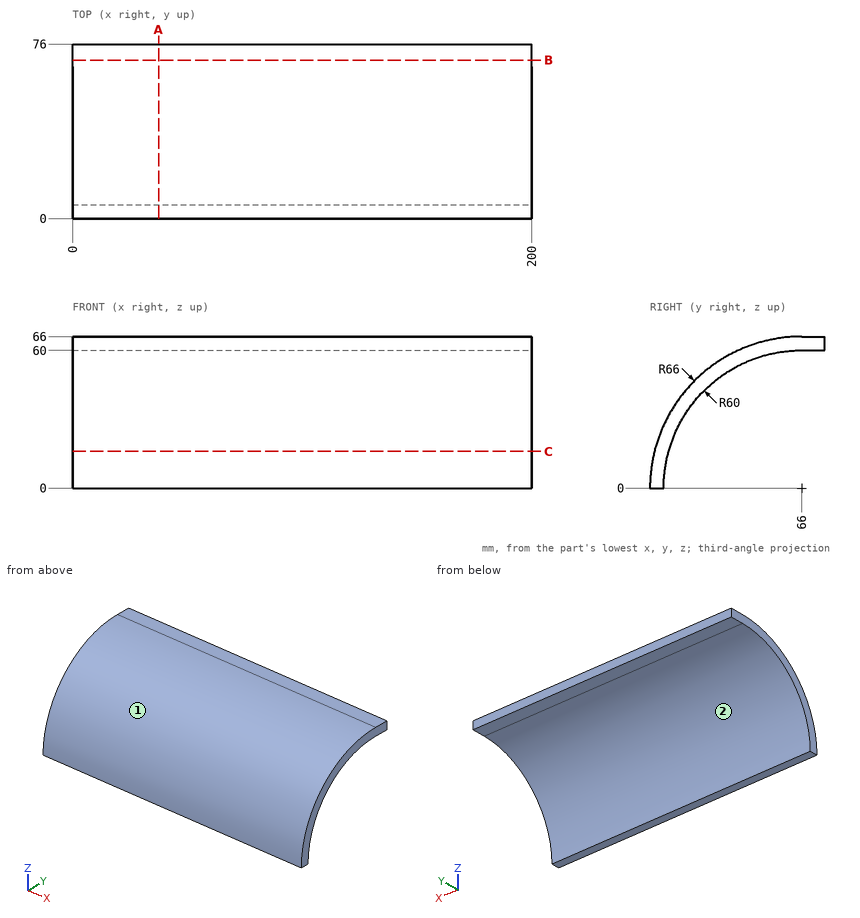
Verification items for this drawing (mm, ordinates from the low corner). Coordinates: 2 decimals unless noted, no trailing zeros. Loops run counter-clockwise (first coordinate to the right, second up) from the corner with the lowest first, then second, coordinate; pieces in that order, holes last. Notation, with made-up numbers: (83, 73) - (129, 73) arc R37 ccw to (129, 111) - close; hole circle Ø2 at (3.5, 13.5). An arc over 180 degrees is marked (long way). Use one line per item in the form item = value. Start each with the question number.
Item 1: Mould release check, pull along Z, two halves, no side actions. Record for the marked faces 1 and 2: +Z half, -Z half, draft (parallel to the pull), parting line (faces both ways), or undercut.
Item 2: Section check A-A, the plane x = 37.5. Enter the section's corners in (y, z).
Item 3: Thickness scan on probe 1 along Z at (x, y) = (176, 64); probe 2 along Z at (x, y) = (65, 25); probe 3 along Y at (x, z) = (47, 34.5) (3 decimals). Record the ranges inside material, lowest first.
Item 4: Section check B-B, the plane y = 69. Enter the section's corners in (x, z), and give its area (3 significant figures).
Item 5: Section check C-C, the plane z = 16. Enter the section's corners in (x, y).
Item 6: Gauge pin test, flat ends, axial feed: pin 1 (3 mm diameter, centred on x = 80, z = 38, fed in from +Y); pin 2 (5 mm diameter, centred on x = 119, y = 69, fed in from -Z); pin 3 (8 mm diameter, centred on x = 168.5, z = 55.5, fed in from -Y). Record the tip position at first contact, or that the pin passes through.
Computed:
q1.face_1 = +Z half
q1.face_2 = -Z half
q2.outline = (0, 0) - (6, 0) arc R60 cw to (66, 60) - (76, 60) - (76, 66) - (66, 66) arc R66 ccw to start
q3.probe_1 = 59.97 to 65.97
q3.probe_2 = 43.81 to 51.72
q3.probe_3 = 9.735 to 16.911
q4.outline = (0, 60) - (200, 60) - (200, 66) - (0, 66) - close
q4.area = 1,200 mm2
q5.outline = (0, 1.97) - (200, 1.97) - (200, 8.17) - (0, 8.17) - close
q6.pin_1 = 20.84
q6.pin_2 = 60
q6.pin_3 = 24.72
